```python
from build123d import *

# Parameters (mm, degrees)
BOSS_EXTRUDE1_DEPTH        = 6.35
F_10_CLEARANCE_HOLE1_D     = 4.9784
F_10_CLEARANCE_HOLE1_DEPTH = 135.89
F_10_CLEARANCE_HOLE1_TIP   = 1.495662253
SKETCH4_R                  = 56
CUT_EXTRUDE1_DEPTH         = 7.35
F_10_CLEARANCE_HOLE2_D     = 5.1054
CIRPATTERN1_COUNT          = 3
CIRPATTERN1_ANGLE          = 120


with BuildPart() as part:
    # Sketch1 → Boss-Extrude1 (new body)
    with BuildSketch(Plane.XY):
        Polygon((-75, 48), (-18.024996339, 85), (-5, 85), (-5, 0), (-75, 0), align=None)
    extrude(amount=BOSS_EXTRUDE1_DEPTH)

    # #10 Clearance Hole1
    with Locations(Plane(origin=(0, 0, 0), x_dir=(-1, 0, 0), z_dir=(0, 0, -1))):
        with Locations((20.435878863, 77.755724401), (67.401430668, 47.25593844)):
            Hole(F_10_CLEARANCE_HOLE1_D / 2, depth=F_10_CLEARANCE_HOLE1_DEPTH)
            with Locations((0, 0, -(F_10_CLEARANCE_HOLE1_DEPTH + F_10_CLEARANCE_HOLE1_TIP / 2))):  # 118° drill point
                Cone(0, F_10_CLEARANCE_HOLE1_D / 2, F_10_CLEARANCE_HOLE1_TIP, mode=Mode.SUBTRACT)

    # Sketch4 → Cut-Extrude1 (cut, through all)
    with BuildSketch(Plane(origin=(0, 0, 0), x_dir=(-1, 0, 0), z_dir=(0, 0, -1))):
        Circle(SKETCH4_R)
    extrude(amount=-CUT_EXTRUDE1_DEPTH, mode=Mode.SUBTRACT)

    # Mirror1: part across plane


with BuildPart() as part_1:
    add(part.part)
    add(part.part.mirror(Plane.ZX))

    # #10 Clearance Hole2 (through all)
    with Locations(Plane.XY.offset(6.35)):
        with Locations((-30, 51.961524227)):
            f_10_clearance_hole2 = Hole(F_10_CLEARANCE_HOLE2_D / 2)

    # CirPattern1: #10 Clearance Hole2 ×3 about axis
    cirpattern1_axis = Axis((0, 0, 0), (0, 0, 1))
    for i in range(1, CIRPATTERN1_COUNT):
        add(f_10_clearance_hole2.rotate(cirpattern1_axis, i * CIRPATTERN1_ANGLE / (CIRPATTERN1_COUNT - 1)), mode=Mode.SUBTRACT)


solid = part_1.part
```
Build history of the part. All positions in model axes, mm. Round coordinates to 2 decimals unless told otherwise and drop trailing zeros. Order: outer loops, then holes, each group sorted by start corner. A loop starts at its lowest first (then second) coordinate and runs counter-clockwise, first axis right, second up. Notation, with made-up numbers: (36.25, -37) -> (58.25, -37) arc R29 cw to (58.25, -11) -> close; hole circle Ø5 at (79.5, 9). An arc over 180 degrees is marked (long way). Answer in a Markdown table with one row per item.
1) Band-saw the part on C-C on x = -41.5. Give the cut face in (y, z), and give its area (3 significant figures).
Values:
| item | result |
|---|---|
| outline | (-69.76, 0) -> (-37.6, 0) -> (-37.6, 6.35) -> (-69.76, 6.35) -> close; (37.6, 0) -> (69.76, 0) -> (69.76, 6.35) -> (37.6, 6.35) -> close |
| area | 408 mm2 |
2) Band-saw the part on B-B on z = 2.5. Give the cut face in (x, y) (3 decimals), and give its area (3 significant figures).
Values:
| item | result |
|---|---|
| outline | (-75, -48) -> (-18.025, -85) -> (-5, -85) -> (-5, -55.776) arc R56 cw to (-5, 55.776) -> (-5, 85) -> (-18.025, 85) -> (-75, 48) -> close; hole circle Ø4.978 at (-67.401, -47.256); hole circle Ø4.978 at (-67.401, 47.256); hole circle Ø5.105 at (-60, 0); hole circle Ø5.105 at (-30, -51.962); hole circle Ø5.105 at (-30, 51.962); hole circle Ø4.978 at (-20.436, -77.756); hole circle Ø4.978 at (-20.436, 77.756) |
| area | 5,290 mm2 |
3) Wall check: L1, parallel to Y at x = -28.5, z = 1.25; L2, parallel to Y at x = -24.5, z = 3; L3, parallel to X at y = -78, z = 6.25. Give the ranges that are in metal, low to high.
Values:
| item | result |
|---|---|
| L1 | -78.2 to -54.03, -49.9 to -48.21, 48.21 to 49.9, 54.03 to 78.2 |
| L2 | -80.8 to -50.36, 50.36 to 80.8 |
| L3 | -28.8 to -22.91, -17.96 to -5 |
4) Band-saw the part on A-A on y = 0. Give the cut face in (x, z), and give its area (3 significant figures).
Values:
| item | result |
|---|---|
| outline | (-75, 0) -> (-62.55, 0) -> (-62.55, 6.35) -> (-75, 6.35) -> close; (-57.45, 0) -> (-56, 0) -> (-56, 6.35) -> (-57.45, 6.35) -> close |
| area | 88.2 mm2 |
5) Pin check, flat tips, straight feed: P1, Ø6, axis at x = -18.5, y = 59, coming from the -Z side; P2, Ø4.5, axis at x = -60, y = 0, coming from the +Z side; P3, Ø2, axis at x = -53, z = 3, coming from the +Y side. Stop position of each tip, or through.
Values:
| item | result |
|---|---|
| P1 | z = 0 |
| P2 | through |
| P3 | y = 62.94 |
6) Mould opens along X. For faces 1 (the flat face through (-5, -71, 3)), 2 (the flat face through (-12, 85, 3)), 3 (the cylindrical face through (-62.55, -0.11, 3.13)) say: released by +X, released by -X, zero draft, split by the parting line, or undercut.
Values:
| item | result |
|---|---|
| face 1 | released by +X |
| face 2 | zero draft |
| face 3 | undercut |
7) Band-saw the part on D-D on y = 71. Give the cut face in (x, z), and give its area (3 significant figures).
Values:
| item | result |
|---|---|
| outline | (-39.58, 0) -> (-5, 0) -> (-5, 6.35) -> (-39.58, 6.35) -> close |
| area | 220 mm2 |
